Build history of the part. All positions in model axes, mm. Round coordinates to 2 decimals unless told otherwise and drop trailing zeros. Loops run counter-clockwise (first coordinate to the right, second up) from the corner with the lowest first, then second, coordinate; pieces in that order, holes last. Notation, with made-up numbers: (-2.75, -29.75) - (11.25, -29.75) arc R19 cw to (11.25, -21.75) - close; hole circle Ø6 at (74.25, 80.5). An arc over 180 degrees is marked (long way). Use a Markdown table: item, result.
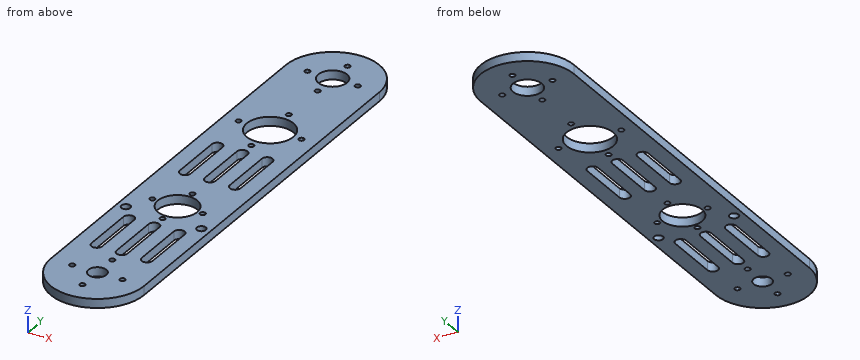
from build123d import *

# Parameters (mm, degrees)
SKETCH_1_R      = 5
SKETCH_1_R_2    = 1.5
SKETCH_1_R_3    = 8
SKETCH_1_R_4    = 2.5
SKETCH_1_R_5    = 13
SKETCH_1_R_6    = 11
EXTRUDE_1_DEPTH = 5


with BuildPart() as part:
    # 草图1 → 凸台-拉伸1 (new body)
    with BuildSketch(Plane.XY):
        with BuildLine():
            Line((-26, 220), (-26, 0))
            ThreePointArc((-26, 0), (0, -26), (26, 0))
            Line((26, 0), (26, 220))
            ThreePointArc((26, 220), (0, 246), (-26, 220))
        make_face()
        Circle(SKETCH_1_R, mode=Mode.SUBTRACT)
        with Locations((0, -14)):
            Circle(SKETCH_1_R_2, mode=Mode.SUBTRACT)
        with Locations(Location((0, 220, 0), (0, 0, 180))):
            Circle(SKETCH_1_R_3, mode=Mode.SUBTRACT)
        with Locations((-14, 0)):
            Circle(SKETCH_1_R_2, mode=Mode.SUBTRACT)
        with Locations((0, 14)):
            Circle(SKETCH_1_R_2, mode=Mode.SUBTRACT)
        with Locations((14, 0)):
            Circle(SKETCH_1_R_2, mode=Mode.SUBTRACT)
        with Locations((-21, 62)):
            Circle(SKETCH_1_R_4, mode=Mode.SUBTRACT)
        with Locations((21, 62)):
            Circle(SKETCH_1_R_4, mode=Mode.SUBTRACT)
        with Locations((0, 89)):
            Circle(SKETCH_1_R_2, mode=Mode.SUBTRACT)
        with Locations((0, 161.5)):
            Circle(SKETCH_1_R_5, mode=Mode.SUBTRACT)
        with Locations((0, 75)):
            Circle(SKETCH_1_R_6, mode=Mode.SUBTRACT)
        with Locations((0, 234)):
            Circle(SKETCH_1_R_2, mode=Mode.SUBTRACT)
        with Locations((14, 220)):
            Circle(SKETCH_1_R_2, mode=Mode.SUBTRACT)
        with Locations((0, 206)):
            Circle(SKETCH_1_R_2, mode=Mode.SUBTRACT)
        with Locations((-14, 220)):
            Circle(SKETCH_1_R_2, mode=Mode.SUBTRACT)
        with Locations((0, 179)):
            Circle(SKETCH_1_R_2, mode=Mode.SUBTRACT)
        with Locations((17.5, 161.5)):
            Circle(SKETCH_1_R_2, mode=Mode.SUBTRACT)
        with Locations((0, 144)):
            Circle(SKETCH_1_R_2, mode=Mode.SUBTRACT)
        with Locations((-17.5, 161.5)):
            Circle(SKETCH_1_R_2, mode=Mode.SUBTRACT)
        with Locations((14, 75)):
            Circle(SKETCH_1_R_2, mode=Mode.SUBTRACT)
        with Locations((0, 61)):
            Circle(SKETCH_1_R_2, mode=Mode.SUBTRACT)
        with Locations((-14, 75)):
            Circle(SKETCH_1_R_2, mode=Mode.SUBTRACT)
        with BuildLine():
            Line((-3, 105.5), (-3, 135.5))
            ThreePointArc((-3, 135.5), (0, 138.5), (3, 135.5))
            Line((3, 135.5), (3, 105.5))
            ThreePointArc((3, 105.5), (0, 102.5), (-3, 105.5))
        make_face(mode=Mode.SUBTRACT)
        with BuildLine():
            Line((-3, 23.001218935), (-3, 53.001218935))
            ThreePointArc((-3, 53.001218935), (0, 56.001218935), (3, 53.001218935))
            Line((3, 53.001218935), (3, 23.001218935))
            ThreePointArc((3, 23.001218935), (0, 20.001218935), (-3, 23.001218935))
        make_face(mode=Mode.SUBTRACT)
        with BuildLine():
            Line((-17, 23.001218935), (-17, 53.001218935))
            ThreePointArc((-17, 53.001218935), (-14, 56.001218935), (-11, 53.001218935))
            Line((-11, 53.001218935), (-11, 23.001218935))
            ThreePointArc((-11, 23.001218935), (-14, 20.001218935), (-17, 23.001218935))
        make_face(mode=Mode.SUBTRACT)
        with BuildLine():
            Line((17, 23.001218935), (17, 53.001218935))
            ThreePointArc((17, 53.001218935), (14, 56.001218935), (11, 53.001218935))
            Line((11, 53.001218935), (11, 23.001218935))
            ThreePointArc((11, 23.001218935), (14, 20.001218935), (17, 23.001218935))
        make_face(mode=Mode.SUBTRACT)
        with BuildLine():
            Line((-16.913638667, 105.5), (-16.913638667, 135.5))
            ThreePointArc((-16.913638667, 135.5), (-13.913638667, 138.5), (-10.913638667, 135.5))
            Line((-10.913638667, 135.5), (-10.913638667, 105.5))
            ThreePointArc((-10.913638667, 105.5), (-13.913638667, 102.5), (-16.913638667, 105.5))
        make_face(mode=Mode.SUBTRACT)
        with BuildLine():
            Line((16.913638667, 105.5), (16.913638667, 135.5))
            ThreePointArc((16.913638667, 135.5), (13.913638667, 138.5), (10.913638667, 135.5))
            Line((10.913638667, 135.5), (10.913638667, 105.5))
            ThreePointArc((10.913638667, 105.5), (13.913638667, 102.5), (16.913638667, 105.5))
        make_face(mode=Mode.SUBTRACT)
    extrude(amount=EXTRUDE_1_DEPTH)


solid = part.part
Q1. Drop flat-ended pins along their axis: pin 1 (1.5 mm diameter, centred on x = -15, z = 1, fed in from +Y); pin 2 (6 mm diameter, centred on x = 0, y = 0, fed in from +Z); pin 3 (1.5 mm diameter, centred on x = -16.5, z = 4, fed in from +Y); pin 4 (3.5 mm diameter, centred on x = 14, y = 0, fed in from +Z). Give the stop position or say it passes through.
Results found:
| item | result |
|---|---|
| pin 1 | stops at y = 241.75 |
| pin 2 | passes through |
| pin 3 | stops at y = 240.69 |
| pin 4 | stops at z = 5 |
Q2. Probe line 1 (X direction, y = 45.5, z = 1.05); line 2 (X direction, y = 220, z = 1.65); line 3 (Y direction, x = -14, z = 1.95). List the from-to ranges inside material, lowest first.
Results found:
| item | result |
|---|---|
| line 1 | x = -26 to -17, -11 to -3, 3 to 11, 17 to 26 |
| line 2 | x = -26 to -15.5, -12.5 to -8, 8 to 12.5, 15.5 to 26 |
| line 3 | y = -21.91 to -1.5, 1.5 to 20, 56 to 73.5, 76.5 to 102.5, 138.5 to 218.5, 221.5 to 241.91 |
Q3. Cut at B-B, the plane z = 3.3. Count the separate pieces of the cut face and the enclosed holes in it, plus the area to 3 significant figures.
Results found:
| item | result |
|---|---|
| separate pieces | 1 |
| enclosed holes | 28 |
| area | 11,000 mm2 |
Q4. Cut at A-A, the plane y = 120. List the corners of the cut face in (x, z), plus the area to 3 significant figures.
Results found:
| item | result |
|---|---|
| outline | (-26, 0) - (-16.91, 0) - (-16.91, 5) - (-26, 5) - close; (-10.91, 0) - (-3, 0) - (-3, 5) - (-10.91, 5) - close; (3, 0) - (10.91, 0) - (10.91, 5) - (3, 5) - close; (16.91, 0) - (26, 0) - (26, 5) - (16.91, 5) - close |
| area | 170 mm2 |
